from build123d import *

# Parameters (mm, degrees)
BOSS_EXTRUDE1_DEPTH      = 10
BOSS_EXTRUDE1_DEPTH_BACK = 3.9
SKETCH2_W                = 6.445
SKETCH2_H                = 4.032
SKETCH2_W_2              = 4.545
SKETCH2_H_2              = 2.132
SKETCH3_W                = 5.745
SKETCH3_H                = 3.332
CUT_EXTRUDE1_DEPTH       = 10
FILLET1_R                = 0.4
BOSS_EXTRUDE2_DEPTH      = 2
BOSS_EXTRUDE2_DEPTH_BACK = 2
CUT_EXTRUDE2_REACH       = 13.831


with BuildPart() as part:
    # Sketch2 → Boss-Extrude1 (new, two sides: drawn at the far end of the back side and taken through both)
    with BuildSketch(Plane.XY.offset(-BOSS_EXTRUDE1_DEPTH_BACK)):
        Rectangle(SKETCH2_W, SKETCH2_H)
        Rectangle(SKETCH2_W_2, SKETCH2_H_2, mode=Mode.SUBTRACT)
    extrude(amount=BOSS_EXTRUDE1_DEPTH + BOSS_EXTRUDE1_DEPTH_BACK)

    # Sketch3 → Cut-Extrude1 (cut)
    with BuildSketch(Plane.XY):
        Rectangle(SKETCH3_W, SKETCH3_H)
    extrude(amount=CUT_EXTRUDE1_DEPTH, mode=Mode.SUBTRACT)

    # Fillet1
    fillet1_edges = [part.edges().sort_by_distance(p)[0] for p in [
        (-3.2225, 2.016, 3.05),
        (3.2225, 2.016, 3.05),
        (3.2225, -2.016, 3.05),
        (-3.2225, -2.016, 3.05),
    ]]
    fillet(fillet1_edges, radius=FILLET1_R)

    # Sketch6 → Boss-Extrude2 (add, two sides: drawn at the far end of the back side and taken through both)
    with BuildSketch(Plane(origin=(0, 0, 0), x_dir=(0, 0, -1), z_dir=(1, 0, 0)).offset(-BOSS_EXTRUDE2_DEPTH_BACK)):
        Polygon((3.9, 2.016), (3.9001, 3.416), (1.339853874, 3.416), (-0.11724349, 3.726), (-1.1, 3.726), (-1.1, 3.326), (-5.098455185, 3.40488658), (-5.098455185, 2.699069635), (-0.216775103, 2.616), (2.605304601, 2.616), (2.605304601, 2.016), align=None)
    extrude(amount=BOSS_EXTRUDE2_DEPTH + BOSS_EXTRUDE2_DEPTH_BACK)

    # Cut-Extrude2: up to this plane
    cut_extrude2_end = Plane(origin=(-2, 2.699069635, 5.098455185), z_dir=(0, -0.9998552489648911, 0.017014144626037273))
    # Sketch7 → Cut-Extrude2 (cut, up to the surface)
    with BuildSketch(Plane(origin=(0, 3.303012132, -0.065166), x_dir=(1, 0, 0), z_dir=(0, 0.9998054348584555, -0.019725425914151256)), mode=Mode.PRIVATE) as cut_extrude2_sk1:
        Polygon((-1, -5.164626041), (-1.3, -1.165392745), (-2, -1.173282915), (-2, -5.164626041), align=None)
    cut_extrude2_tool1 = split(extrude(cut_extrude2_sk1.sketch, amount=-CUT_EXTRUDE2_REACH, mode=Mode.PRIVATE), bisect_by=cut_extrude2_end, keep=Keep.BOTH, mode=Mode.PRIVATE)
    add(cut_extrude2_tool1.solids().sort_by_distance((-1.570429, 3.367797, 3.218548))[0], mode=Mode.SUBTRACT)
    # Sketch7 → Cut-Extrude2 (cut, up to the surface)
    with BuildSketch(Plane(origin=(0, 3.303012132, -0.065166), x_dir=(1, 0, 0), z_dir=(0, 0.9998054348584555, -0.019725425914151256)), mode=Mode.PRIVATE) as cut_extrude2_sk2:
        Polygon((1, -5.164626041), (1.3, -1.165392745), (2, -1.173282915), (2, -5.164626041), align=None)
    cut_extrude2_tool2 = split(extrude(cut_extrude2_sk2.sketch, amount=-CUT_EXTRUDE2_REACH, mode=Mode.PRIVATE), bisect_by=cut_extrude2_end, keep=Keep.BOTH, mode=Mode.PRIVATE)
    add(cut_extrude2_tool2.solids().sort_by_distance((1.570429, 3.367797, 3.218548))[0], mode=Mode.SUBTRACT)


solid = part.part
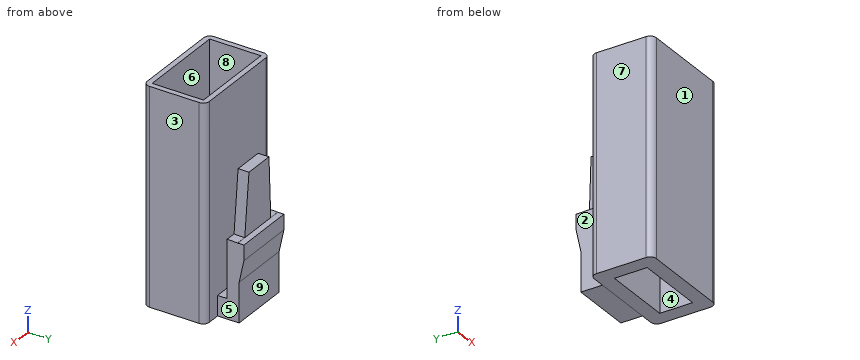
The listing builds one solid part. Answer for the finished solid, in the listing's coordinates (mm). Face numbers are marked on the shaded views. A direction names the side the tool comes from. Give positions to 0.01 mm unless a question says otherwise; leave off trailing zeros. Order: outer loops, then holes, each group sorted by start corner. A loop starts at its lowest first (then second) coordinate and runs counter-clockwise, first axis right, second up. Notation, with made-up numbers: (-30, 72) - (13, 72) arc R4 ccw to (13, 76) - close; hole circle Ø9 at (49, 78). An arc over 180 degrees is marked (long way). One line per item, written item: value. Start each with the question number.
1) A cutting plane is placed at D-D on z = 5.75. Give the vertices of the cut face in (x, y).
2) A cutting plane is placed at A-A on x = -0.5. Give the vertices of the cut face in (y, z), then the cut area to 3 significant figures.
3) Find the intervals of material crossed by L1, parallel to X at y = 1.5, z = 2.25; L2, parallel to X at y = -0.6, z = -3.25; L3, parallel to Y at x = 2, z = 5.25, in increasing order.
4) A cutting plane is placed at B-B on z = 4.25. Give the vertices of the cut face in (x, y).
5) The mould has two halves that part along Y. Classify the marked faces 6, 7, 8 and 9: released by +Y, released by -Y, zero draft, split by the parting line, or undercut.
6) A cutting plane is placed at C-C on y = -0.6. Give the vertices of the cut face in (x, z).
7) A tool of negligible diameter and unlimited length cuts with its end or side. For the marked faces 1, 2, 3, 4 and 5, from which of +Z, -Z, +X, -X, +Y, -Y can it reach the whole face along a straight path? Write none if from no direction.
8) Given pin 1 Ø3 at (x, z) = (0, 4) entering from +Y; pin 2 Ø0.9 at (y, z) = (2.5, -1.5) entering from -X; pin 3 Ø1.4 at (y, z) = (3, -2) entering from +X, each flat-ended and moving along its own axis, determine where each tip first touches the part or whether it passes through.
Answer sheet:
1. outline: (-3.22, -1.62) arc R0.4 ccw to (-2.82, -2.02) - (2.82, -2.02) arc R0.4 ccw to (3.22, -1.62) - (3.22, 1.62) arc R0.4 ccw to (2.82, 2.02) - (-2.82, 2.02) arc R0.4 ccw to (-3.22, 1.62) - close; hole (-2.87, -1.67) - (2.87, -1.67) - (2.87, 1.67) - (-2.87, 1.67) - close
2. outline: (-2.02, -3.9) - (-1.07, -3.9) - (-1.07, 0) - (-1.67, 0) - (-1.67, 10) - (-2.02, 10) - close; (1.07, -3.9) - (2.02, -3.9) - (3.42, -3.9) - (3.42, -1.34) - (3.73, 0.12) - (3.73, 1.1) - (3.33, 1.1) - (3.4, 5.1) - (2.7, 5.1) - (2.62, 0.22) - (2.62, -2.61) - (2.02, -2.61) - (2.02, 10) - (1.67, 10) - (1.67, 0) - (1.07, 0) - close
2. area: 22.5 mm2
3. L1: x = -3.22 to -2.87, 2.87 to 3.22
3. L2: x = -3.22 to -2.27, 2.27 to 3.22
3. L3: y = -2.02 to -1.67, 1.67 to 2.02
4. outline: (-3.22, -1.62) arc R0.4 ccw to (-2.82, -2.02) - (2.82, -2.02) arc R0.4 ccw to (3.22, -1.62) - (3.22, 1.62) arc R0.4 ccw to (2.82, 2.02) - (-2.82, 2.02) arc R0.4 ccw to (-3.22, 1.62) - close; (-1.06, 2.68) - (1.06, 2.68) - (1.06, 3.39) - (-1.06, 3.39) - close; hole (-2.87, -1.67) - (2.87, -1.67) - (2.87, 1.67) - (-2.87, 1.67) - close
5. face 6: undercut
5. face 7: zero draft
5. face 8: undercut
5. face 9: released by +Y
6. outline: (-3.22, -3.9) - (-2.27, -3.9) - (-2.27, 0) - (-2.87, 0) - (-2.87, 10) - (-3.22, 10) - close; (2.27, -3.9) - (3.22, -3.9) - (3.22, 10) - (2.87, 10) - (2.87, 0) - (2.27, 0) - close
7. face 1: +Z, -Z, +X, -X, -Y
7. face 2: +Z, -Z, -X, +Y
7. face 3: +Z, -Z, +X, +Y, -Y
7. face 4: +Z, -Z
7. face 5: +Z, -Z, +X, +Y
8. pin 1: stops at y = 3.4
8. pin 2: stops at x = -2
8. pin 3: stops at x = 2
